Verification items for the finished model (mm, model axes). Face numbers are marked on the shaded views. Coordinates: 2 decimals unless noted, no trailing zeros. Order: outer loops, then holes, each group sorted by start corner. A loop starts at its lowest first (then second) coordinate and runs counter-clockwise, first axis right, second up. Notation, with made-up numbers: M -19,23 L -15,23 A24 cw -15,59 Z; hole C 58,25.5 d1. An arc over 180 degrees is marked long. Use one line per item in the form item = value. Start each with the question number.
Autodesk Inventor part; units mm, degrees
ref_plane "YZ Plane" through (0, 0, 0) normal (1, 0, 0) x (0, 1, 0)
ref_plane "XZ Plane" through (0, 0, 0) normal (0, 1, 0) x (-1, 0, 0)
ref_plane "XY Plane" through (0, 0, 0) normal (0, 0, 1) x (1, 0, 0)
sketch "Sketch1" plane through (0, 0, 0) normal (0, 0, 1) x (1, 0, 0)
  circle A0 centre (0, 0) radius 5
  arc A1 (-13, 15) -> (-15, 13) centre (-13, 13) ccw
  arc A2 (-15, -13) -> (-13, -15) centre (-13, -13) ccw
  arc A3 (13, -15) -> (15, -13) centre (13, -13) ccw
  arc A4 (15, 13) -> (13, 15) centre (13, 13) ccw
  arc A5 (-13, 14) -> (-14, 13) centre (-13, 13) ccw
  arc A6 (-14, -13) -> (-13, -14) centre (-13, -13) ccw
  arc A7 (13, -14) -> (14, -13) centre (13, -13) ccw
  arc A8 (14, 13) -> (13, 14) centre (13, 13) ccw
  line L0 (14, -14) -> (-14, 14) construction
  line L1 (-14, -14) -> (14, 14) construction
  line L2 (15, -15) -> (-15, 15) construction
  line L3 (-15, -15) -> (15, 15) construction
  line L4 (-13, 15) -> (-8, 15)
  line L5 (-8, 13) -> (-8, 8) construction
  line L6 (-9.4142, 8) -> (-13, 8)
  line L7 (-15, 8) -> (-15, 13)
  line L8 (-13, -15) -> (-8, -15)
  line L9 (-8, -13) -> (-8, -9.4142)
  line L10 (-9.4142, -8) -> (-13, -8)
  line L11 (-15, -8) -> (-15, -13)
  line L12 (13, -15) -> (8, -15)
  line L13 (8, -13) -> (8, -9.4142)
  line L14 (9.4142, -8) -> (13, -8)
  line L15 (15, -8) -> (15, -13)
  line L16 (13, 15) -> (8, 15)
  line L17 (8, 13) -> (8, 9.4142)
  line L18 (9.4142, 8) -> (13, 8)
  line L19 (15, 8) -> (15, 13)
  line L20 (-13, 9) -> (-10, 9)
  line L21 (-9, 10) -> (-9, 13)
  line L22 (-10, 14) -> (-13, 14)
  line L23 (-14, 13) -> (-14, 10)
  line L24 (13, 9) -> (10, 9)
  line L25 (9, 10) -> (9, 13)
  line L26 (10, 14) -> (13, 14)
  line L27 (14, 13) -> (14, 10)
  line L28 (13, -9) -> (10, -9)
  line L29 (9, -10) -> (9, -13)
  line L30 (10, -14) -> (13, -14)
  line L31 (14, -13) -> (14, -10)
  line L32 (-13, -9) -> (-10, -9)
  line L33 (-9, -10) -> (-9, -13)
  line L34 (-10, -14) -> (-13, -14)
  line L35 (-14, -13) -> (-14, -10)
  line L36 (-14, 13) -> (-14, 10)
  line L37 (-14, -10) -> (-14, -13)
  line L38 (-14, -13) -> (-14, -10)
  line L39 (-14, 10) -> (-14, 13)
  line L40 (13, -15) -> (5, -15)
  line L41 (-5, -15) -> (-13, -15)
  line L42 (13, -15) -> (5, -15) construction
  line L43 (0, -15) -> (-13, -15) construction
  line L44 (4, -13) -> (8, -13)
  line L45 (-8, -13) -> (-4, -13)
  line L46 (10, -9) -> (13, -9)
  line L47 (14, -10) -> (14, -13)
  line L48 (13, -14) -> (10, -14)
  line L49 (9, -13) -> (9, -10)
  line L50 (5, -14) -> (5, -15)
  line L51 (13, -14) -> (10, -14)
  line L52 (5, -14) -> (4, -14)
  line L53 (4, -14) -> (5, -14)
  line L54 (10, -14) -> (13, -14)
  line L55 (-4, -14) -> (-5, -14)
  line L56 (-10, -14) -> (-13, -14)
  line L57 (-13, -14) -> (-10, -14)
  line L58 (-5, -14) -> (-4, -14)
  line L59 (14, -13) -> (14, -10)
  line L60 (14, 10) -> (14, 13)
  line L61 (14, 13) -> (14, 10)
  line L62 (14, -10) -> (14, -13)
  line L63 (-5, -14) -> (-5, -15)
  line L64 (10, 14) -> (13, 14)
  line L65 (13, 14) -> (10, 14)
  line L66 (-10, 14) -> (-13, 14)
  line L67 (-13, 14) -> (-10, 14)
  line L68 (-5, 15) -> (-5, 14)
  line L69 (-13, 15) -> (-5, 15)
  line L70 (5, 15) -> (13, 15)
  line L71 (-15, 15) -> (-5, 15) construction
  line L72 (5, 15) -> (15, 15) construction
  line L73 (5, 15) -> (5, 14)
  line L74 (8, 13) -> (4, 13)
  line L75 (5, 14) -> (4, 14)
  line L76 (-5, 14) -> (-4, 14)
  line L77 (4, 14) -> (5, 14)
  line L78 (-4, 13) -> (-8, 13)
  line L79 (-4, 14) -> (-5, 14)
  line L80 (4, 13) -> (4, 14)
  line L81 (-4, 13) -> (-4, 14)
  line L82 (-4, -14) -> (-4, -13)
  line L83 (4, -14) -> (4, -13)
  line L84 (-8, 9.4142) -> (-4.1919, 5.6061)
  line L85 (8, 9.4142) -> (4.1919, 5.6061)
  line L86 (9.4142, 8) -> (5.6061, 4.1919)
  line L87 (5.6061, -4.1919) -> (9.4142, -8)
  line L88 (4.1919, -5.6061) -> (8, -9.4142)
  line L89 (-4.1919, -5.6061) -> (-8, -9.4142)
  line L90 (-5.6061, -4.1919) -> (-9.4142, -8)
  line L91 (-9.4142, 8) -> (-5.6061, 4.1919)
  arc A9 (4.1919, 5.6061) -> (-4.1919, 5.6061) centre (0, 0) ccw
  arc A10 (5.6061, -4.1919) -> (5.6061, 4.1919) centre (0, 0) ccw
  arc A11 (-5.6061, 4.1919) -> (-5.6061, -4.1919) centre (0, 0) ccw
  arc A12 (-4.1919, -5.6061) -> (4.1919, -5.6061) centre (0, 0) ccw
  line L92 (-8, 13) -> (-8, 9.4142)
  line L93 (-15, -13) -> (-15, -5) construction
  line L94 (-15, -13) -> (-15, -5)
  line L95 (-15, 5) -> (-15, 13)
  line L96 (15, -5) -> (15, -13) construction
  line L97 (15, 13) -> (15, 5)
  line L98 (15, -5) -> (15, -13)
  line L99 (-14, -4) -> (-14, -5)
  line L100 (14, -4) -> (14, -5)
  line L101 (14, 4) -> (14, 5)
  line L102 (-14, 4) -> (-14, 5)
  line L103 (-13, 8) -> (-13, 4)
  line L104 (13, 4) -> (13, 8)
  line L105 (13, -8) -> (13, -4)
  line L106 (-13, -4) -> (-13, -8)
  line L107 (-14, -5) -> (-15, -5)
  line L108 (15, -5) -> (14, -5)
  line L109 (15, 5) -> (14, 5)
  line L110 (-14, 5) -> (-15, 5)
  line L111 (13, 4) -> (14, 4)
  line L112 (-14, 4) -> (-13, 4)
  line L113 (-14, -4) -> (-13, -4)
  line L114 (13, -4) -> (14, -4)
  arc A13 (-13, -9) -> (-14, -10) centre (-13, -10) ccw
  arc A14 (-9, -10) -> (-10, -9) centre (-10, -10) ccw
  arc A15 (-10, -14) -> (-9, -13) centre (-10, -13) ccw
  arc A16 (10, -9) -> (9, -10) centre (10, -10) ccw
  arc A17 (9, -13) -> (10, -14) centre (10, -13) ccw
  arc A18 (14, -10) -> (13, -9) centre (13, -10) ccw
  arc A19 (10, 14) -> (9, 13) centre (10, 13) ccw
  arc A20 (9, 10) -> (10, 9) centre (10, 10) ccw
  arc A21 (13, 9) -> (14, 10) centre (13, 10) ccw
  arc A22 (-9, 13) -> (-10, 14) centre (-10, 13) ccw
  arc A23 (-10, 9) -> (-9, 10) centre (-10, 10) ccw
  arc A24 (-14, 10) -> (-13, 9) centre (-13, 10) ccw
  point P0 (15, -15)
  point P1 (-5.5858, -7)
  dimension "d0" = 30
  dimension "d1" = 30
  dimension "d2" = 10
  dimension "d4" = 2
  dimension "d11" = 28
  dimension "d12" = 7
  dimension "d13" = 7
  dimension "d15" = 1
  dimension "d16" = 1
  dimension "d17" = 1
  dimension "d18" = 1
  dimension "d19" = 5
  dimension "d23" = 30
  dimension "d27" = 1
  dimension "d30" = 3.5858
  dimension "d31" = 2
  dimension "d32" = 16
  dimension "d33" = 8
  dimension "d34" = 6
  dimension "d35" = 5.5858
extrude "Extrusion1" add sketch "Sketch1" along normal mid plane 105.1
sketch "Sketch3" plane through (-13, -15, 52.55) normal (0, -1, 0) x (1, 0, 0)
  line L0 (18, -105.1) -> (8, -105.1)
  line L1 (0, -105.1) -> (-1, -105.1)
  line L2 (-1, -105.1) -> (0, -105.1)
  line L3 (0, -105.1) -> (3, -105.1)
  line L4 (3, -105.1) -> (4, -105.1)
  line L5 (4, -105.1) -> (3, -105.1)
  line L6 (3, -105.1) -> (0, -105.1)
  line L7 (26, -105.1) -> (23, -105.1)
  line L8 (23, -105.1) -> (22, -105.1)
  line L9 (22, -105.1) -> (23, -105.1)
  line L10 (23, -105.1) -> (26, -105.1)
  line L11 (26, -105.1) -> (27, -105.1)
  line L12 (27, -105.1) -> (26, -105.1)
  line L13 (4, -105.1) -> (3, -105.1)
  line L14 (3, -105.1) -> (0, -105.1)
  line L15 (0, -105.1) -> (-1, -105.1)
  line L16 (-1, -105.1) -> (0, -105.1)
  line L17 (0, -105.1) -> (3, -105.1)
  line L18 (3, -105.1) -> (4, -105.1)
  line L19 (23, -105.1) -> (22, -105.1)
  line L20 (22, -105.1) -> (23, -105.1)
  line L21 (23, -105.1) -> (26, -105.1)
  line L22 (26, -105.1) -> (27, -105.1)
  line L23 (27, -105.1) -> (26, -105.1)
  line L24 (26, -105.1) -> (23, -105.1)
  line L25 (5, -105.1) -> (8.8081, -105.1)
  line L26 (8.8081, -105.1) -> (17.1919, -105.1)
  line L27 (17.1919, -105.1) -> (21, -105.1)
  line L28 (21, -105.1) -> (17, -105.1)
  line L29 (17, -105.1) -> (18, -105.1)
  line L30 (18, -105.1) -> (26, -105.1)
  line L31 (26, -105.1) -> (28, -105.1)
  line L32 (28, -105.1) -> (27, -105.1)
  line L33 (27, -105.1) -> (26, -105.1)
  line L34 (26, -105.1) -> (22.4142, -105.1)
  line L35 (22.4142, -105.1) -> (18.6061, -105.1)
  line L36 (18.6061, -105.1) -> (18.6061, -105.1)
  line L37 (18.6061, -105.1) -> (22.4142, -105.1)
  line L38 (22.4142, -105.1) -> (26, -105.1)
  line L39 (26, -105.1) -> (27, -105.1)
  line L40 (27, -105.1) -> (28, -105.1)
  line L41 (28, -105.1) -> (26, -105.1)
  line L42 (26, -105.1) -> (18, -105.1)
  line L43 (18, -105.1) -> (17, -105.1)
  line L44 (17, -105.1) -> (21, -105.1)
  line L45 (21, -105.1) -> (17.1919, -105.1)
  line L46 (17.1919, -105.1) -> (8.8081, -105.1)
  line L47 (8.8081, -105.1) -> (5, -105.1)
  line L48 (5, -105.1) -> (9, -105.1)
  line L49 (9, -105.1) -> (8, -105.1)
  line L50 (8, -105.1) -> (0, -105.1)
  line L51 (0, -105.1) -> (-2, -105.1)
  line L52 (-2, -105.1) -> (-1, -105.1)
  line L53 (-1, -105.1) -> (0, -105.1)
  line L54 (0, -105.1) -> (3.5858, -105.1)
  line L55 (3.5858, -105.1) -> (7.3939, -105.1)
  line L56 (7.3939, -105.1) -> (7.3939, -105.1)
  line L57 (7.3939, -105.1) -> (3.5858, -105.1)
  line L58 (3.5858, -105.1) -> (0, -105.1)
  line L59 (0, -105.1) -> (-1, -105.1)
  line L60 (-1, -105.1) -> (-2, -105.1)
  line L61 (-2, -105.1) -> (0, -105.1)
  line L62 (0, -105.1) -> (8, -105.1)
  line L63 (8, -105.1) -> (9, -105.1)
  line L64 (9, -105.1) -> (5, -105.1)
  line L65 (39.4927, -113.2765) -> (-27.442, -65.6557)
  line L66 (-27.442, -65.6557) -> (-27.442, -113.2765)
  line L67 (27, -105.1) -> (27, 0)
  line L68 (-27.442, -113.2765) -> (39.4927, -113.2765)
  point P0 (13, -52.55)
  dimension "d36" = 35.43
extrude "Extrusion2" cut sketch "Sketch3" against normal blind 30
properties part number "pole_supoort_2" material "Aluminum 6061"
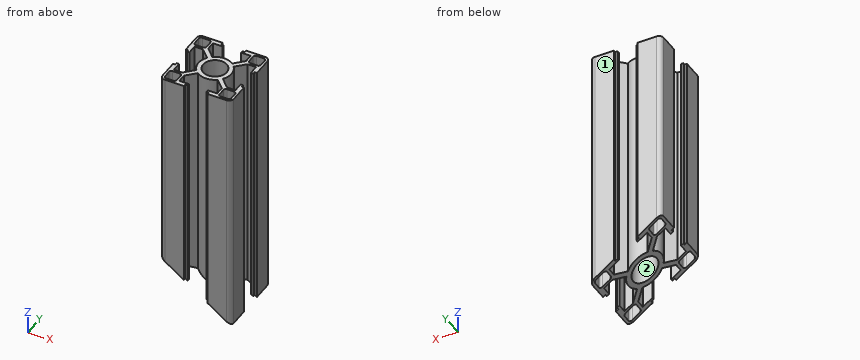
1. Cross-section at A-A on y = -11.75. Enter the section's corners in (x, z), and give its area (3 significant figures).
2. Cross-section at D-D on z = -8. Give the number of separate pieces and of enclosed holes in the cut face, and give its area (3 significant figures).
3. Cross-section at C-C on y = -1.5. Enter the section's corners in (x, z), and give its area (3 significant figures).
4. Depth check by flat-ended pin: P1, Ø0.5, axis at x = 14.5, z = -16.5, coming from the -Y side; P2, Ø12, axis at x = -4.5, y = 9.5, coming from the -Z side; P3, Ø2, axis at x = 0, z = -24.5, coming from the +Y side. Enter the tip coordinate at first touch or a pass-through.
5. Cross-section at B-B on x = 0. Enter the section's corners in (y, z).
6. Release check for a two-part mould opening along X. For the marked faces 1 and 2 record: pulls with the +X half, pulls with the -X half, needs draft (parallel to the pull), parting line crosses it, or undercut.
7. Material ranges on line 1 along X through (y, z) = (-11.5, -21); line 2 along X through (y, z) = (0, -22.5), recorded low to high.
Final values:
q1.outline = M -15,-31.21 L -14,-31.92 L -14,52.55 L -15,52.55 Z; M -9,-35.48 L -8,-36.19 L -8,52.55 L -9,52.55 Z; M 8,-47.57 L 9,-48.28 L 9,52.55 L 8,52.55 Z; M 14,-51.84 L 15,-52.55 L 15,52.55 L 14,52.55 Z
q1.area = 378 mm2
q2.separate_pieces = 1
q2.enclosed_holes = 5
q2.area = 266 mm2
q3.outline = M -6.84,-37.01 L -4.77,-38.48 L -4.77,52.55 L -6.84,52.55 Z; M 4.77,-45.27 L 6.84,-46.74 L 6.84,52.55 L 4.77,52.55 Z
q3.area = 391 mm2
q4.P1 = -14.56
q4.P2 = -42.54
q4.P3 = 7
q5.outline = M -7,-41.88 L -5,-41.88 L -5,52.55 L -7,52.55 Z; M 5,-41.88 L 7,-41.88 L 7,52.55 L 5,52.55 Z
q6.face_1 = needs draft
q6.face_2 = undercut
q7.line_1 = -15 to -14, -9 to -8, 8 to 9, 14 to 15
q7.line_2 = -7 to -5, 5 to 7
